The model under review builds one solid part; all positions refer to its coordinate system, in mm. Face numbers are marked on the shaded views. Coordinates: 2 decimals unless noted, no trailing zeros. Write each loop counter-clockwise with the first axis right and the second up, starting at its lowest first coordinate (ties: lowest second). Pieces come first, ordered by that corner, then holes. Notation, with made-up numbers: (35.5, 56) - (49.5, 56) arc R37 cw to (49.5, 92) - close; hole circle Ø11 at (3, 47). An arc over 180 degrees is marked (long way). Use one line per item in the form item = value. Start each with the question number.
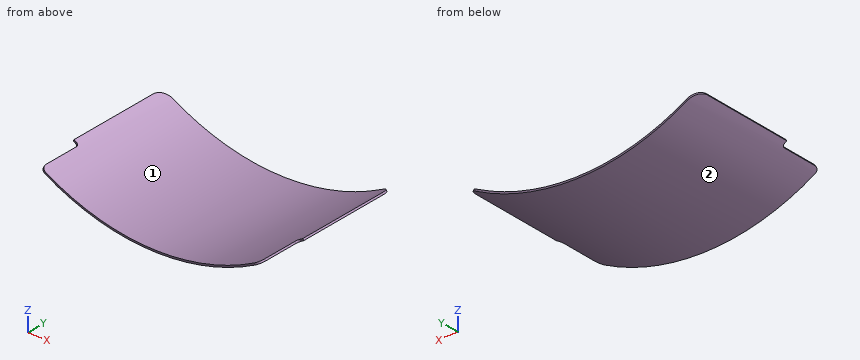
```python
from build123d import *

# Parameters (mm, degrees)
EXTRUS_O_FINA1_DEPTH   = 125
ESBO_O3_W              = 10
ESBO_O3_H              = 75
CORTE_EXTRUS_O1_DEPTH  = 10
FILETE5_R              = 5
FILETE6_R              = 20
FILETE5_OF_ESPELHAR6_R = 5
FILETE8_R              = 10


with BuildPart() as part:
    # Esboço2 → Extrusão-Fina1 (new, symmetric)
    with BuildSketch(Plane(origin=(0, 0, 0), x_dir=(1, 0, 0), z_dir=(0, 1, 0))):
        with BuildLine():
            ThreePointArc((-194.216199756, -56.278928136), (0, -1.5), (194.216199756, -56.278928136))
            Line((194.216199756, -56.278928136), (195.783800244, -53.721071864))
            ThreePointArc((195.783800244, -53.721071864), (0, 1.5), (-195.783800244, -53.721071864))
            Line((-195.783800244, -53.721071864), (-194.216199756, -56.278928136))
        make_face()
    extrude(amount=EXTRUS_O_FINA1_DEPTH, both=True)

    # Esboço3 → Corte-extrusão1 (cut)
    with BuildSketch(Plane(origin=(166.260657734, 0, 101.894031669), x_dir=(0.5225334957369068, 0, -0.8526187576126673), z_dir=(0.8526187576126673, 0, 0.5225334957369068))):
        with Locations((55.5, -87.5)):
            Rectangle(ESBO_O3_W, ESBO_O3_H)
    corte_extrus_o1 = extrude(amount=-CORTE_EXTRUS_O1_DEPTH, mode=Mode.SUBTRACT)

    # Filete5
    filete5_edges = [part.edges().sort_by_distance(p)[0] for p in [
        (186.403788141, -50, 49.888923779),
    ]]
    fillet(filete5_edges, radius=FILETE5_R)

    # Filete6
    filete6_edges = [part.edges().sort_by_distance(p)[0] for p in [
        (-195, 125, 55),
        (195, 125, 55),
    ]]
    fillet(filete6_edges, radius=FILETE6_R)

    # Espelhar6: Corte-extrusão1 across plane
    add(corte_extrus_o1.mirror(Plane(origin=(0, 0, 0), x_dir=(0, 0, 1), z_dir=(1, 0, 0))), mode=Mode.SUBTRACT)

    # Filete5 of Espelhar6
    filete5_of_espelhar6_edges = [part.edges().sort_by_distance(p)[0] for p in [
        (-186.403788141, -50, 49.888923779),
    ]]
    fillet(filete5_of_espelhar6_edges, radius=FILETE5_OF_ESPELHAR6_R)

    # Filete8
    filete8_edges = [part.edges().sort_by_distance(p)[0] for p in [
        (186.403788141, -125, 49.888923779),
        (-186.403788141, -125, 49.888923779),
    ]]
    fillet(filete8_edges, radius=FILETE8_R)


solid = part.part
```
1. Take a section at B-B (y = -7). State the section outline as (x, z) points, plus the area to 3 significant figures.
2. Take a section at A-A (z = 28). State the section outline as (x, y) points.
3. For L1, parallel to X at y = 9, z = 40.5; L2, parallel to X at y = 53, z = 49; L3, parallel to Z at x = -80.5, y = -34.5, list the stretches that pass through material, from the lowest coordinate up.
4. For P1, Ø5, axis at x = -90, y = 24, coming from the -Z side; P2, Ø3, axis at y = 56.5, z = 39, coming from the -X side; P3, Ø6, axis at x = -55.5, y = -1, coming from the -Z side, all flat-tipped, find the tip position at first contact; note any pin that passes through.
5. Take a section at C-C (z = 10). State the section outline as (x, y) points.
6. The part is to be moulded in two halves that separate along X. For the marked faces 1 and 2, say which applies: released by +X, released by -X, zero draft, split by the parting line, or undercut.
Returned:
q1.outline = (-195.78, 53.72) arc R374.68 ccw to (195.78, 53.72) - (194.22, 56.28) arc R371.68 cw to (-194.22, 56.28) - close
q1.area = 1,230 mm²
q2.outline = (-145.73, -125) - (-137.83, -125) - (-137.83, 125) - (-145.73, 125) - close; (137.83, -125) - (145.73, -125) - (145.73, 125) - (137.83, 125) - close
q3.L1 = -172.36 to -165.74, 165.74 to 172.36
q3.L2 = -187.86 to -181.81, 181.81 to 187.86
q3.L3 = 7.25 to 10.32
q4.P1 = 8.86
q4.P2 = -172.36
q4.P3 = 2.2
q5.outline = (-92.12, -125) - (-79.03, -125) - (-79.03, 125) - (-92.12, 125) - close; (79.03, -125) - (92.12, -125) - (92.12, 125) - (79.03, 125) - close
q6.face_1 = undercut
q6.face_2 = split by the parting line
